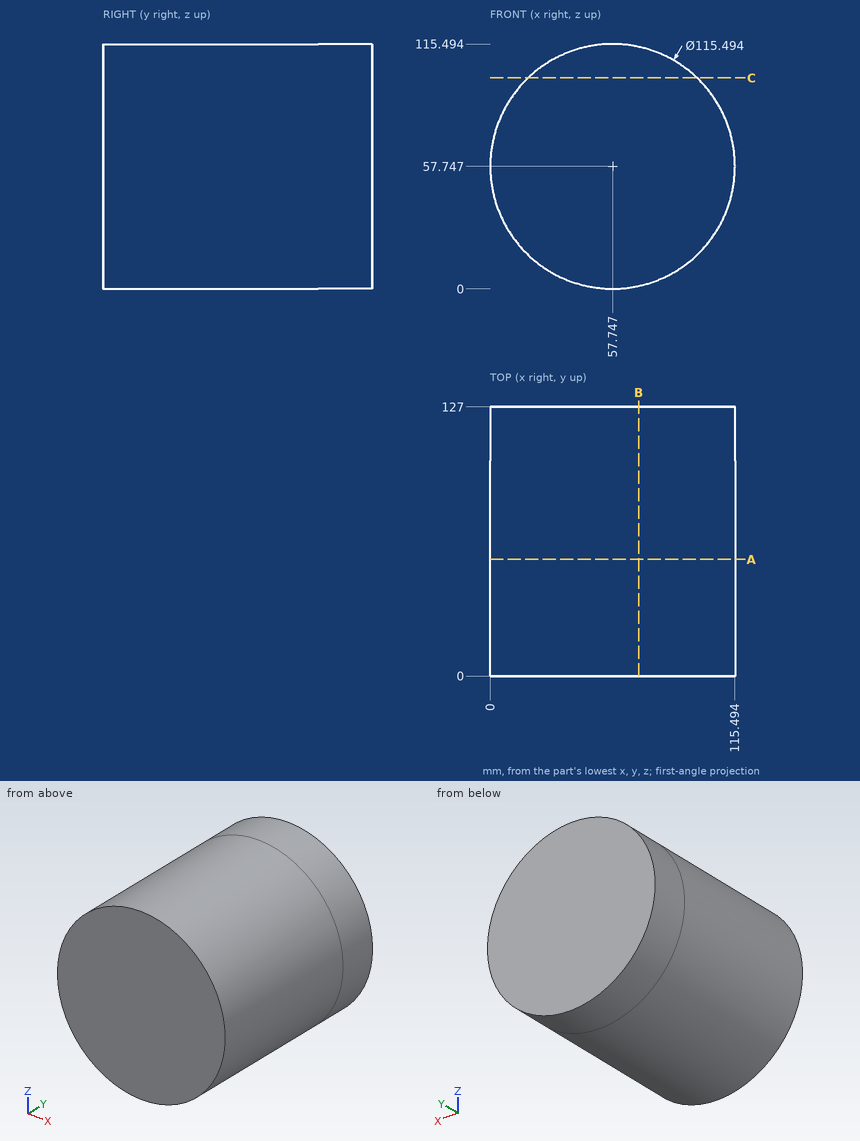
Geometry: see drawing. Coordinates: mm, zero at the bounding-box minimum. Coordinates: 2 decimals unless noted, no trailing zeros. Order: outer loops, then holes, each group sorted by start corner. A loop starts at its lowest first (then second) coordinate and runs counter-clockwise, first axis right, second up. Notation, with made-up numbers: (35.5, 65) - (71.5, 65) arc R24 cw to (71.5, 96) - close; hole circle Ø7 at (12, -35). An arc over 180 degrees is marked (long way). Write each question's results on one line, items separated by ' | '.
(1) Section query B-B, the plane x = 70. Return the cut outline in (y, z) (1 decimal).
Values found:
outline: (0, 1.3) - (127, 1.3) - (127, 114.2) - (0, 114.2) - close
(2) Section query C-C, the plane z = 99.5. Return the cut outline in (x, y) (1 decimal), plus the area to 3 significant figures.
Values found:
outline: (17.9, 0) - (97.6, 0) - (97.6, 127) - (17.9, 127) - close | area: 10,100 mm²
(3) First-contact query: pin 1 Ø6 at (x, y) = (98, 58.5) entering from -Z; pin 2 Ø8 at (y, z) = (104, 99.5) entering from +X (1 decimal); pin 3 Ø12 at (x, y) = (60.5, 32.5) entering from +Z (1 decimal). Flat tips, straight axial feed; report the tip coordinate or a pass-through.
Values found:
pin 1: stops at z = 13.62 | pin 2: stops at x = 101.4 | pin 3: stops at z = 115.5
(4) Line query: line 1 (X direction, y = 111, z = 58); line 2 (Z direction, x = 57, y = 67) (1 decimal); line 3 (X direction, y = 61, z = 21) (1 decimal). Output: solid intervals per line, ascending. Write a range as [from, to].
Values found:
line 1: x = [0, 115.49] | line 2: z = [0, 115.5] | line 3: x = [13.2, 102.3]
(5) Section query A-A, the plane y = 55. Return the cut outline in (x, z) (1 decimal), plus the area to 3 significant figures.
Values found:
outline: circle Ø115.5 at (57.7, 57.7) | area: 10,500 mm²
